```python
from build123d import *

# Parameters (mm, degrees)
MODEL_R                 = 1.5
SALIENTE_EXTRUIR1_DEPTH = 3
CROQUIS1_W              = 6.3
CROQUIS1_H              = 6.3
CORTAR_EXTRUIR1_DEPTH   = 2


with BuildPart() as part:
    # Model → Saliente-Extruir1 (new body)
    with BuildSketch(Plane.XY):
        with BuildLine():
            Line((64.337531364, 275.445982488), (61.837531364, 277.945982488))
            Line((61.837531364, 277.945982488), (61.837531364, 283.629591549))
            ThreePointArc((61.837531364, 283.629591549), (61.338785756, 285.688708663), (59.953103236, 287.29139217))
            Line((59.953103236, 287.29139217), (52.511010495, 292.607172698))
            ThreePointArc((52.511010495, 292.607172698), (51.268737063, 293.230701866), (49.895438624, 293.445372078))
            Line((49.895438624, 293.445372078), (25.779624104, 293.445372078))
            ThreePointArc((25.779624104, 293.445372078), (24.406325665, 293.230701866), (23.164052233, 292.607172698))
            Line((23.164052233, 292.607172698), (15.721959492, 287.29139217))
            ThreePointArc((15.721959492, 287.29139217), (14.336276972, 285.688708663), (13.837531364, 283.629591549))
            Line((13.837531364, 283.629591549), (13.837531364, 277.945982488))
            Line((13.837531364, 277.945982488), (11.337531364, 275.445982488))
            Line((11.337531364, 275.445982488), (10.837531364, 275.445982488))
            ThreePointArc((10.837531364, 275.445982488), (6.337531364, 270.945982488), (10.837531364, 266.445982488))
            Line((10.837531364, 266.445982488), (10.837531364, 248.445982488))
            ThreePointArc((10.837531364, 248.445982488), (6.337531364, 243.945982488), (10.837531364, 239.445982488))
            Line((10.837531364, 239.445982488), (11.337531364, 239.445982488))
            Line((11.337531364, 239.445982488), (13.837531364, 236.945982488))
            Line((13.837531364, 236.945982488), (13.837531364, 231.261763016))
            ThreePointArc((13.837531364, 231.261763016), (14.336276972, 229.202645903), (15.721959492, 227.599962396))
            Line((15.721959492, 227.599962396), (23.164052233, 222.284181867))
            ThreePointArc((23.164052233, 222.284181867), (24.406325665, 221.660652699), (25.779624104, 221.445982488))
            Line((25.779624104, 221.445982488), (49.895438624, 221.445982488))
            ThreePointArc((49.895438624, 221.445982488), (51.268737063, 221.660652699), (52.511010495, 222.284181867))
            Line((52.511010495, 222.284181867), (59.953103236, 227.599962396))
            ThreePointArc((59.953103236, 227.599962396), (61.338785756, 229.202645903), (61.837531364, 231.261763016))
            Line((61.837531364, 231.261763016), (61.837531364, 236.945982488))
            Line((61.837531364, 236.945982488), (64.337531364, 239.445982488))
            Line((64.337531364, 239.445982488), (64.837531364, 239.445982488))
            ThreePointArc((64.837531364, 239.445982488), (69.337531364, 243.945982488), (64.837531364, 248.445982488))
            Line((64.837531364, 248.445982488), (64.837531364, 266.445982488))
            ThreePointArc((64.837531364, 266.445982488), (69.337531364, 270.945982488), (64.837531364, 275.445982488))
            Line((64.837531364, 275.445982488), (64.337531364, 275.445982488))
        make_face()
        with Locations((28.837531364, 225.945982488)):
            Circle(MODEL_R, mode=Mode.SUBTRACT)
        with Locations((10.837531364, 243.945982488)):
            Circle(MODEL_R, mode=Mode.SUBTRACT)
        with BuildLine():
            ThreePointArc((18.092271793, 254.345372089), (14.992271793, 257.445372089), (18.092271793, 260.545372089))
            Line((18.092271793, 260.545372089), (21.737271793, 260.545677294))
            ThreePointArc((21.737271793, 260.545677294), (24.837271793, 257.445677294), (21.737271793, 254.345677294))
            Line((21.737271793, 254.345677294), (18.092271793, 254.345372089))
        make_face(mode=Mode.SUBTRACT)
        with Locations((37.837531364, 225.945982488)):
            Circle(MODEL_R, mode=Mode.SUBTRACT)
        with Locations((46.837531364, 225.945982488)):
            Circle(MODEL_R, mode=Mode.SUBTRACT)
        with Locations((64.837531364, 243.945982488)):
            Circle(MODEL_R, mode=Mode.SUBTRACT)
        with BuildLine():
            ThreePointArc((53.937271793, 254.345677294), (50.837271793, 257.445677294), (53.937271793, 260.545677294))
            Line((53.937271793, 260.545677294), (57.582271793, 260.545372089))
            ThreePointArc((57.582271793, 260.545372089), (60.682141998, 257.445242304), (57.582012214, 254.3453721))
            Line((57.582012214, 254.3453721), (53.937271793, 254.345677294))
        make_face(mode=Mode.SUBTRACT)
        with Locations((10.837531364, 270.945982488)):
            Circle(MODEL_R, mode=Mode.SUBTRACT)
        with Locations((28.837531364, 288.945982488)):
            Circle(MODEL_R, mode=Mode.SUBTRACT)
        with BuildLine():
            Line((18.337531364, 264.945372078), (18.337531364, 275.445372078))
            ThreePointArc((18.337531364, 275.445372078), (20.973570333, 281.809333109), (27.337531364, 284.445372078))
            Line((27.337531364, 284.445372078), (48.337531364, 284.445372078))
            ThreePointArc((48.337531364, 284.445372078), (54.701492395, 281.809333109), (57.337531364, 275.445372078))
            Line((57.337531364, 275.445372078), (57.337531364, 264.945372078))
            ThreePointArc((57.337531364, 264.945372078), (56.898191536, 263.884711906), (55.837531364, 263.445372078))
            Line((55.837531364, 263.445372078), (53.998048837, 263.445372078))
            Line((53.998048837, 263.445372078), (53.877013891, 263.445372078))
            ThreePointArc((53.877013891, 263.445372078), (47.939939639, 257.615658143), (53.537303053, 251.459040723))
            Line((53.537303053, 251.459040723), (55.837531364, 251.459040723))
            ThreePointArc((55.837531364, 251.459040723), (56.898191536, 251.019700895), (57.337531364, 249.959040723))
            Line((57.337531364, 249.959040723), (57.337531364, 239.445982488))
            ThreePointArc((57.337531364, 239.445982488), (54.701492395, 233.082021457), (48.337531364, 230.445982488))
            Line((48.337531364, 230.445982488), (27.337531364, 230.445982488))
            ThreePointArc((27.337531364, 230.445982488), (20.973570333, 233.082021457), (18.337531364, 239.445982488))
            Line((18.337531364, 239.445982488), (18.337531364, 249.959040723))
            ThreePointArc((18.337531364, 249.959040723), (18.776871192, 251.019700895), (19.837531364, 251.459040723))
            Line((19.837531364, 251.459040723), (22.137759676, 251.459040723))
            ThreePointArc((22.137759676, 251.459040723), (27.735123089, 257.615658143), (21.798048837, 263.445372078))
            Line((21.798048837, 263.445372078), (21.677013891, 263.445372078))
            Line((21.677013891, 263.445372078), (19.837531364, 263.445372078))
            ThreePointArc((19.837531364, 263.445372078), (18.776871192, 263.884711906), (18.337531364, 264.945372078))
        make_face(mode=Mode.SUBTRACT)
        with Locations((64.837531364, 270.945982488)):
            Circle(MODEL_R, mode=Mode.SUBTRACT)
        with Locations((37.837531364, 288.945982488)):
            Circle(MODEL_R, mode=Mode.SUBTRACT)
        with Locations((46.837531364, 288.945982488)):
            Circle(MODEL_R, mode=Mode.SUBTRACT)
    extrude(amount=SALIENTE_EXTRUIR1_DEPTH)

    # Croquis1 → Cortar-Extruir1 (cut)
    with BuildSketch(Plane.XY.offset(3)):
        with Locations((37.837531364, 288.945982488)):
            Rectangle(CROQUIS1_W, CROQUIS1_H)
        with Locations((37.837531364, 225.945982488)):
            Rectangle(CROQUIS1_W, CROQUIS1_H)
    extrude(amount=-CORTAR_EXTRUIR1_DEPTH, mode=Mode.SUBTRACT)


solid = part.part
```
Could you check a few things on this model? Use its own coordinates, in mm. A direction names the side the tool comes from. Round coordinates to 2 decimals unless told otherwise and drop trailing zeros. Loops run counter-clockwise (first coordinate to the right, second up) from the corner with the lowest first, then second, coordinate; pieces in that order, holes last. Notation, with made-up numbers: (7.5, 22) - (65.5, 22) arc R22 cw to (65.5, 40) - close; hole circle Ø11 at (72.25, 75). An arc over 180 degrees is marked (long way). Answer in a Markdown table with one row per item. Add a question column.
(1) I need wall thicknesses on line 1 along Y through (x, z) = (65, 2.65); line 2 along X through (y, z) = (244, 0.8); line 3 along X through (y, z) = (290, 1.85). Which ranges of each line are inside material? Lowest first, please.
(2) I'm going to push flat-ended pins straight in: pin 1 (0.7 mm diameter, centred on x = 21, z = 2, fed in from -Y); pin 2 (1 mm diameter, centred on y = 284, z = 2, fed in from +X); pin 3 (0.6 mm diameter, centred on y = 225, z = 2.5, fed in from -X). Where does each tip first touch, or does it pass through?
(3) If we section it at B-B (y = 238.5): Please give me the cut outline in (x, z), plus the area to 3 significant figures.
(4) If we section it at D-D (z = 0.5): State how many separate pieces and enclosed holes the cut face has, plus the area to 3 significant figures.
(5) For faces 4 (the face through (21, 263.445, 1)), 5 (the face through (34.688, 289, 2)), 6 (the face through (61.838, 234, 1)), 7 (the face through (12.57, 238.213, 1.479)), 8 (the face through (24.425, 293.237, 1.479)), which set-ups out of +Z, -Z, +X, -X, +Y, -Y let a thin tool reach every point of the face, with its end or its side?
(6) If we section it at C-C (y = 268): Please give me the cut outline in (x, z), plus the area to 3 significant figures.
(7) If we mould it in two halves opening along X, with no side actions, what happens to faces 1 (the face through (18.338, 270, 1)), 2 (the face through (10.838, 258, 1)), 3 (the face through (69.336, 243.847, 1.479))? For each: pulls with the +X half, pulls with the -X half, needs draft (parallel to the pull), parting line crosses it, or undercut.
(8) If we section it at A-A (x = 29): Please give me the cut outline in (y, z).
Model answer:
| question | item | result |
|---|---|---|
| 1 | line 1 | y = 239.45 to 242.45, 245.44 to 248.44, 266.45 to 269.45, 272.44 to 275.44 |
| 1 | line 2 | x = 6.34 to 9.34, 12.34 to 18.34, 57.34 to 63.34, 66.34 to 69.34 |
| 1 | line 3 | x = 19.51 to 27.77, 29.9 to 34.69, 40.99 to 45.77, 47.9 to 56.16 |
| 2 | pin 1 | stops at y = 223.58 |
| 2 | pin 2 | stops at x = 61.84 |
| 2 | pin 3 | stops at x = 18.94 |
| 3 | outline | (12.28, 0) - (18.39, 0) - (18.39, 3) - (12.28, 3) - close; (57.29, 0) - (63.39, 0) - (63.39, 3) - (57.29, 3) - close |
| 3 | area | 36.6 mm² |
| 4 | separate pieces | 1 |
| 4 | enclosed holes | 13 |
| 4 | area | 1,630 mm² |
| 5 | face 4 | +Z, -Z |
| 5 | face 5 | +Z |
| 5 | face 6 | +Z, -Z, +X, -Y |
| 5 | face 7 | +Z, -Z, -X, -Y |
| 5 | face 8 | +Z, -Z, -X, +Y |
| 6 | outline | (7.44, 0) - (18.34, 0) - (18.34, 3) - (7.44, 3) - close; (57.34, 0) - (68.24, 0) - (68.24, 3) - (57.34, 3) - close |
| 6 | area | 65.4 mm² |
| 7 | face 1 | undercut |
| 7 | face 2 | pulls with the -X half |
| 7 | face 3 | pulls with the +X half |
| 8 | outline | (221.45, 0) - (224.45, 0) - (224.45, 3) - (221.45, 3) - close; (227.44, 0) - (230.45, 0) - (230.45, 3) - (227.44, 3) - close; (284.45, 0) - (287.45, 0) - (287.45, 3) - (284.45, 3) - close; (290.44, 0) - (293.45, 0) - (293.45, 3) - (290.44, 3) - close |
